Autodesk Inventor part; units mm, degrees
ref_plane "YZ Plane" through (0, 0, 0) normal (1, 0, 0) x (0, 1, 0)
ref_plane "XZ Plane" through (0, 0, 0) normal (0, 1, 0) x (-1, 0, 0)
ref_plane "XY Plane" through (0, 0, 0) normal (0, 0, 1) x (1, 0, 0)
sketch "Sketch1" plane through (0, 0, 0) normal (0, 0, 1) x (1, 0, 0)
  line L0 (0, 0) -> (6.146, 0)
  line L1 (6.4, 0.254) -> (6.4, 0.5)
  line L2 (6.4, 0.5) -> (6.646, 0.5)
  line L3 (6.9, 0.754) -> (6.9, 1.546)
  line L4 (0, 0) -> (0, 6.146)
  line L5 (0.254, 6.4) -> (0.5, 6.4)
  line L6 (0.5, 6.4) -> (0.5, 6.646)
  line L7 (0.754, 6.9) -> (1.5449, 6.9)
  line L8 (1.7989, 6.646) -> (1.7989, 4.8147)
  line L9 (6.646, 1.8) -> (4.754, 1.8)
  line L10 (20, 0) -> (20, 6.146)
  line L11 (19.746, 6.4) -> (19.5, 6.4)
  line L12 (19.5, 6.4) -> (19.5, 6.646)
  line L13 (19.246, 6.9) -> (18.4551, 6.9)
  line L14 (18.2011, 6.646) -> (18.2011, 4.8147)
  line L15 (20, 0) -> (13.854, 0)
  line L16 (13.6, 0.254) -> (13.6, 0.5)
  circle A0 centre (10, 10) radius 2.5
  line L17 (20, 20) -> (13.854, 20)
  line L18 (20, 20) -> (20, 13.854)
  line L19 (19.746, 13.6) -> (19.5, 13.6)
  line L20 (19.5, 13.6) -> (19.5, 13.354)
  line L21 (19.246, 13.1) -> (18.454, 13.1)
  line L22 (13.6, 19.746) -> (13.6, 19.5)
  line L23 (13.6, 19.5) -> (13.354, 19.5)
  line L24 (13.1, 19.246) -> (13.1, 18.454)
  line L25 (13.354, 18.2) -> (15.246, 18.2)
  line L26 (0, 20) -> (6.146, 20)
  line L27 (6.4, 19.746) -> (6.4, 19.5)
  line L28 (6.4, 19.5) -> (6.646, 19.5)
  line L29 (6.9, 19.246) -> (6.9, 18.454)
  line L30 (6.646, 18.2) -> (4.754, 18.2)
  line L31 (0, 20) -> (0, 13.854)
  line L32 (0.254, 13.6) -> (0.5, 13.6)
  line L33 (0.5, 13.6) -> (0.5, 13.354)
  line L34 (0.754, 13.1) -> (1.546, 13.1)
  line L35 (1.8, 13.354) -> (1.8, 15.246)
  line L36 (3.4393, 15.5) -> (2.054, 15.5)
  line L37 (4.5, 16.5607) -> (4.5, 17.946)
  line L38 (16.5, 4.5607) -> (17.9471, 4.5607)
  line L39 (13.6, 0.5) -> (13.354, 0.5)
  line L40 (13.1, 0.754) -> (13.1, 1.546)
  line L41 (13.354, 1.8) -> (15.246, 1.8)
  line L42 (15.5, 2.054) -> (15.5, 3.4393)
  line L43 (15.5, 16.5607) -> (15.5, 17.946)
  line L44 (16.5, 15.4393) -> (17.946, 15.4393)
  line L45 (4.5, 3.4393) -> (4.5, 2.054)
  line L46 (3.5, 4.5607) -> (2.0529, 4.5607)
  line L47 (6.1, 7.6867) -> (6.1, 12.3133)
  line L48 (3.5, 4.5607) -> (5.728, 6.7887)
  line L49 (3.4393, 15.5) -> (5.728, 13.2113)
  line L50 (7.6867, 13.9) -> (12.3133, 13.9)
  line L51 (6.7887, 14.272) -> (4.5, 16.5607)
  line L52 (13.2113, 14.272) -> (15.5, 16.5607)
  line L53 (13.9, 12.3133) -> (13.9, 7.6867)
  line L54 (14.272, 6.7887) -> (16.5, 4.5607)
  line L55 (14.272, 13.2113) -> (16.5, 15.4393)
  line L56 (7.6867, 6.1) -> (12.3133, 6.1)
  line L57 (6.7887, 5.728) -> (4.5, 3.4393)
  line L58 (13.2113, 5.728) -> (15.5, 3.4393)
  arc A1 (6.9, 19.246) -> (6.646, 19.5) centre (6.646, 19.246) ccw
  arc A2 (6.4, 19.746) -> (6.146, 20) centre (6.146, 19.746) ccw
  arc A3 (6.646, 18.2) -> (6.9, 18.454) centre (6.646, 18.454) ccw
  arc A4 (4.754, 18.2) -> (4.5, 17.946) centre (4.754, 17.946) ccw
  arc A5 (13.1, 18.454) -> (13.354, 18.2) centre (13.354, 18.454) ccw
  arc A6 (13.354, 19.5) -> (13.1, 19.246) centre (13.354, 19.246) ccw
  arc A7 (13.854, 20) -> (13.6, 19.746) centre (13.854, 19.746) ccw
  arc A8 (15.5, 17.946) -> (15.246, 18.2) centre (15.246, 17.946) ccw
  arc A9 (2.054, 15.5) -> (1.8, 15.246) centre (2.054, 15.246) ccw
  arc A10 (0.5, 13.354) -> (0.754, 13.1) centre (0.754, 13.354) ccw
  arc A11 (0, 13.854) -> (0.254, 13.6) centre (0.254, 13.854) ccw
  arc A12 (1.546, 13.1) -> (1.8, 13.354) centre (1.546, 13.354) ccw
  arc A13 (0.254, 6.4) -> (0, 6.146) centre (0.254, 6.146) ccw
  arc A14 (0.754, 6.9) -> (0.5, 6.646) centre (0.754, 6.646) ccw
  arc A15 (1.7989, 6.646) -> (1.5449, 6.9) centre (1.5449, 6.646) ccw
  arc A16 (1.7989, 4.8147) -> (2.0529, 4.5607) centre (2.0529, 4.8147) ccw
  arc A17 (19.746, 13.6) -> (20, 13.854) centre (19.746, 13.854) ccw
  arc A18 (19.246, 13.1) -> (19.5, 13.354) centre (19.246, 13.354) ccw
  arc A19 (18.2, 13.354) -> (18.454, 13.1) centre (18.454, 13.354) ccw
  line L59 (18.2, 13.354) -> (18.2, 15.1853)
  arc A20 (18.2, 15.1853) -> (17.946, 15.4393) centre (17.946, 15.1853) ccw
  arc A21 (20, 6.146) -> (19.746, 6.4) centre (19.746, 6.146) ccw
  arc A22 (19.5, 6.646) -> (19.246, 6.9) centre (19.246, 6.646) ccw
  arc A23 (18.4551, 6.9) -> (18.2011, 6.646) centre (18.4551, 6.646) ccw
  arc A24 (17.9471, 4.5607) -> (18.2011, 4.8147) centre (17.9471, 4.8147) ccw
  arc A25 (13.6, 0.254) -> (13.854, 0) centre (13.854, 0.254) ccw
  arc A26 (13.1, 0.754) -> (13.354, 0.5) centre (13.354, 0.754) ccw
  arc A27 (13.354, 1.8) -> (13.1, 1.546) centre (13.354, 1.546) ccw
  arc A28 (15.246, 1.8) -> (15.5, 2.054) centre (15.246, 2.054) ccw
  arc A29 (6.146, 0) -> (6.4, 0.254) centre (6.146, 0.254) ccw
  arc A30 (6.646, 0.5) -> (6.9, 0.754) centre (6.646, 0.754) ccw
  arc A31 (6.9, 1.546) -> (6.646, 1.8) centre (6.646, 1.546) ccw
  arc A32 (4.5, 2.054) -> (4.754, 1.8) centre (4.754, 2.054) ccw
  arc A33 (6.7887, 14.272) -> (7.6867, 13.9) centre (7.6867, 15.17) ccw
  arc A34 (12.3133, 13.9) -> (13.2113, 14.272) centre (12.3133, 15.17) ccw
  arc A35 (6.1, 12.3133) -> (5.728, 13.2113) centre (4.83, 12.3133) ccw
  arc A36 (5.728, 6.7887) -> (6.1, 7.6867) centre (4.83, 7.6867) ccw
  arc A37 (7.6867, 6.1) -> (6.7887, 5.728) centre (7.6867, 4.83) ccw
  arc A38 (13.2113, 5.728) -> (12.3133, 6.1) centre (12.3133, 4.83) ccw
  arc A39 (13.9, 7.6867) -> (14.272, 6.7887) centre (15.17, 7.6867) ccw
  arc A40 (14.272, 13.2113) -> (13.9, 12.3133) centre (15.17, 12.3133) ccw
  point P0 (20, 6.4)
  point P1 (19.5, 6.9)
  point P2 (18.2011, 6.9)
  dimension "d59" = 1.27
extrude "Extrusion1" add sketch "Sketch1" along normal blind 100
properties part number "T slot beam 20mm Dist_40mm"
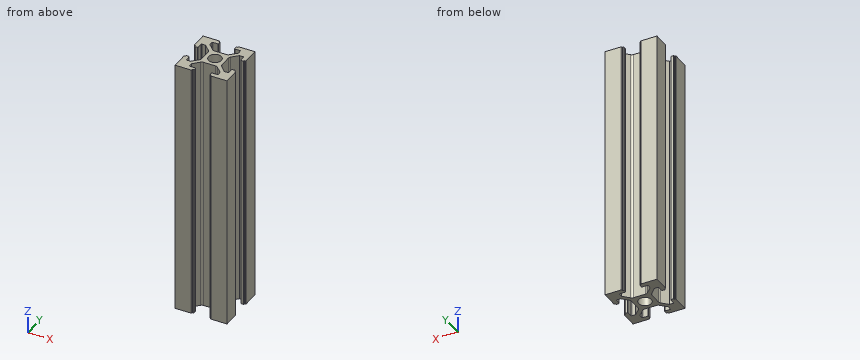
Here's how the part is built. I have some questions about the finished solid (model axes, mm). Coordinates: 2 decimals unless noted, no trailing zeros. Write each loop counter-clockwise with the first axis right and the second up, starting at its lowest first coordinate (ties: lowest second). Pieces come first, ordered by that corner, then holes. Notation, with made-up numbers: M 16,83.25 L 28,83.25 A30 cw 28,122.25 Z; hole C 44,73.25 d7. An arc over 180 degrees is marked long. Answer as CSV lines item,"result". Start each with the question number.
Q1. I need wall thicknesses on probe 1 along X at (y, z) = (1, 78); probe 2 along X at (y, z) = (5.5, 19). Which ranges of each line are inside material? Lowest first, please. Write a range as [from, to].
Q2. Suppose I cut it at A-A, the plane x = 10. List the corners of the cut face in (y, z) for me, then the cut area to 3 significant figures.
Q3. Will these pins go through, and if not, where does the flat tip stop? pin 1 Ø5 at (x, z) = (9, 52) entering from -Y; pin 2 Ø6 at (y, z) = (10, 34) entering from -X.
Entries:
1,probe 1,"x = [0, 6.9], [13.1, 20]"
1,probe 2,"x = [0, 1.8], [4.44, 6.56], [13.44, 15.56], [18.2, 20]"
2,outline,"M 6.1,0 L 7.5,0 L 7.5,100 L 6.1,100 Z; M 12.5,0 L 13.9,0 L 13.9,100 L 12.5,100 Z"
2,area,"280 mm²"
3,pin 1,"stops at y = 0.5"
3,pin 2,"stops at x = 5.9"
